Part model, mm, in its own coordinate system. Face numbers are marked on the shaded views. A direction names the side the tool comes from. Round coordinates to 2 decimals unless told otherwise and drop trailing zeros. Loops run counter-clockwise (first coordinate to the right, second up) from the corner with the lowest first, then second, coordinate; pieces in that order, holes last. Notation, with made-up numbers: M 64,13.5 L 123,13.5 A27 ccw 123,39.5 Z; hole C 5.5,70.5 d5. An arc over 180 degrees is marked long. Put each result on its own line as item: value. Start each with the question number.
1) Drop flat-ended pins along their axis: pin 1 Ø8.5 at (x, y) = (21.5, 27) entering from -Z; pin 2 Ø5 at (x, y) = (6.5, 29) entering from -Z; pin 3 Ø2 at (x, z) = (10, -1) entering from -Y. Give the stop position or say it passes through.
2) Pull direction X, two halves, no side cores. Call the marked faces 3, 4 and 5: +X half, -X half, draft (parallel to the pull), parting line (faces both ways), or undercut.
3) Probe line 1 along X through (y, z) = (22.5, 1.45); line 2 along Y through (x, z) = (8, 1.4). List the from-to ranges inside material, lowest first.
4) Slice it at D-D on y = 12. Give the cut face in (x, z), then the cut area to 3 significant figures.
5) Slice it at C-C on x = 20.5. Give the cut face in (y, z), then the cut area to 3 significant figures.
6) Slice it at B-B on z = -1. Give the cut face in (x, y), then the cut area to 3 significant figures.
7) Which spindle directions (+Z, -Z, +X, -X, +Y, -Y) get a long thin tool onto all of the face, cutting with end or side? Do the marked faces 1 and 2. Say none if no direction does.
8) Slice it at A-A on z = 0.8. Give the cut face in (x, y).
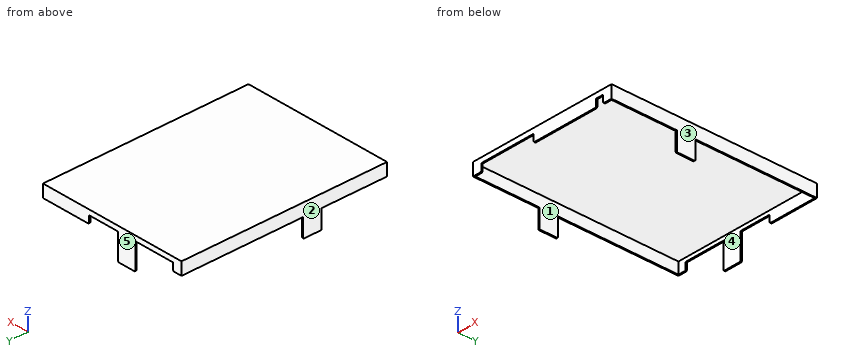
```python
from build123d import *

# Parameters (mm, degrees)
SKETCH_1_W          = 23.9
SKETCH_1_H          = 32.9
EXTRUDE_1_DEPTH     = 2
SHELL_1_T           = -0.2
SKETCH_3_2_W        = 9
SKETCH_3_2_H        = 0.2
SKETCH_3_2_W_2      = 1.2
SKETCH_3_2_W_3      = 5
SKETCH_3_2_W_4      = 6.5
CUT_EXTRUDE_3_DEPTH = 1.2
SKETCH_3_W          = 3
SKETCH_3_H          = 0.2
SKETCH_3_W_2        = 0.2
SKETCH_3_H_2        = 3
EXTRUDE_2_DEPTH     = 3
FILLET_1_R          = 0.2


with BuildPart() as part:
    # Sketch 1 → Extrude 1 (new body)
    with BuildSketch(Plane.XY):
        with Locations((11.8, 16.3)):
            Rectangle(SKETCH_1_W, SKETCH_1_H)
    extrude(amount=EXTRUDE_1_DEPTH)

    # Shell 1
    shell_1_openings = [part.faces().sort_by_distance(p)[0] for p in [
        (11.8, 16.3, 0),
    ]]
    offset(amount=SHELL_1_T, openings=shell_1_openings, kind=Kind.INTERSECTION)

    # Sketch 3_2 → Cut-Extrude 3 (cut)
    with BuildSketch(Plane(origin=(0, 0, 0), x_dir=(-1, 0, 0), z_dir=(0, 0, -1))):
        with Locations((-5.8, -0.05)):
            Rectangle(SKETCH_3_2_W, SKETCH_3_2_H)
        with Locations((-21.7, -0.05)):
            Rectangle(SKETCH_3_2_W_2, SKETCH_3_2_H)
        with Locations((-13.3, 32.65)):
            Rectangle(SKETCH_3_2_W_3, SKETCH_3_2_H)
        with Locations((-4.55, 32.65)):
            Rectangle(SKETCH_3_2_W_4, SKETCH_3_2_H)
    extrude(amount=-CUT_EXTRUDE_3_DEPTH, mode=Mode.SUBTRACT)

    # Sketch 3 → Extrude 2 (add)
    with BuildSketch(Plane(origin=(0, 0, 0), x_dir=(-1, 0, 0), z_dir=(0, 0, -1))):
        with Locations((-9.3, 32.65)):
            Rectangle(SKETCH_3_W, SKETCH_3_H)
        with Locations((-23.65, 11.8)):
            Rectangle(SKETCH_3_W_2, SKETCH_3_H_2)
        with Locations((0.05, 11.8)):
            Rectangle(SKETCH_3_W_2, SKETCH_3_H_2)
    extrude(amount=EXTRUDE_2_DEPTH)

    # Fillet 1
    fillet_1_edges = [part.edges().sort_by_distance(p)[0] for p in [
        (-0.05, 13.3, -3),
        (-0.05, 10.3, -3),
        (23.65, 13.3, -3),
        (23.65, 10.3, -3),
        (1.3, -0.05, 0),
        (10.3, -0.05, 0),
        (21.1, -0.05, 0),
        (22.3, -0.05, 0),
        (15.8, 32.65, 0),
        (1.3, 32.65, 0),
        (7.8, 32.65, -3),
        (10.8, 32.65, -3),
    ]]
    fillet(fillet_1_edges, radius=FILLET_1_R)


solid = part.part
```
Recorded:
1. pin 1: stops at z = 0
1. pin 2: stops at z = 1.8
1. pin 3: stops at y = 32.55
2. face 3: +X half
2. face 4: undercut
2. face 5: draft
3. line 1: x = -0.15 to 0.05, 23.55 to 23.75
3. line 2: y = -0.15 to 0.05, 32.55 to 32.75
4. outline: M -0.15,-3 L 0.05,-3 L 0.05,1.8 L 23.55,1.8 L 23.55,-3 L 23.75,-3 L 23.75,2 L -0.15,2 Z
4. area: 6.70 mm2
5. outline: M -0.15,0 L 0.05,0 L 0.05,1.8 L 32.55,1.8 L 32.55,0 L 32.75,0 L 32.75,2 L -0.15,2 Z
5. area: 7.30 mm2
6. outline: M -0.15,10.3 L 0.05,10.3 L 0.05,13.3 L -0.15,13.3 Z; M 7.8,32.55 L 10.8,32.55 L 10.8,32.75 L 7.8,32.75 Z; M 23.55,10.3 L 23.75,10.3 L 23.75,13.3 L 23.55,13.3 Z
6. area: 1.80 mm2
7. face 1: -Z
7. face 2: +Z, -Z, -X, +Y, -Y
8. outline: M -0.15,-0.15 L 1.3,-0.15 L 1.3,0.05 L 0.05,0.05 L 0.05,32.55 L 1.3,32.55 L 1.3,32.75 L -0.15,32.75 Z; M 7.8,32.55 L 10.8,32.55 L 10.8,32.75 L 7.8,32.75 Z; M 10.3,-0.15 L 21.1,-0.15 L 21.1,0.05 L 10.3,0.05 Z; M 15.8,32.55 L 23.55,32.55 L 23.55,0.05 L 22.3,0.05 L 22.3,-0.15 L 23.75,-0.15 L 23.75,32.75 L 15.8,32.75 Z
